The listing builds one solid part. Answer for the finished solid, in the listing's coordinates (mm). Round coordinates to 2 decimals unless told otherwise and drop trailing zeros. Order: outer loops, then holes, each group sorted by start corner. A loop starts at its lowest first (then second) coordinate and runs counter-clockwise, first axis right, second up. Notation, with made-up numbers: (28, 16.25) -> (50, 16.25) arc R14 ccw to (50, 33.25) -> close; hole circle Ø7 at (-22.5, -13). An arc over 180 degrees is marked (long way). Return JSON: item names as keys, results as strings. Group by question number.
(1) This flat-tipped pin is pushed along its axis until it touches: pin 1 (1.5 mm diameter, centred on y = 0.5, z = 18.5, fed in from +X). Where does it stop, or does it pass through?
(2) The part is cut by section A-A (z = 1). Determine the outline of the cut face in (x, y), plus the area to 3 significant figures.
(3) Consider line 1 (X direction, y = 0.85, z = 10); line 2 (Z direction, x = 26.5, y = 0.85). Determine where each line is inside the solid, lowest interval first. Write a range as [from, to].
(4) The part is cut by section B-B (x = 1). Determine the outline of the cut face in (y, z).
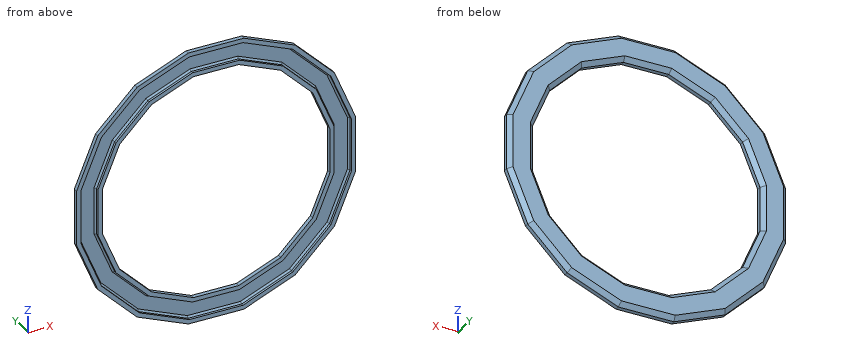
from build123d import *

# Parameters (mm, degrees)
BOSS_EXTRUDE1_DEPTH = 4
CHAMFER1_SIZE       = 2
SHELL1_T            = -2


with BuildPart() as part:
    # Sketch1 → Boss-Extrude1 (new body)
    with BuildSketch(Plane(origin=(0, 0, 0), x_dir=(1, 0, 0), z_dir=(0, 1, 0))):
        Polygon((36.819542328, 55.104339226), (12.92930388, 65), (-12.92930388, 65), (-36.819542328, 55.104339226), (-55.104339226, 36.819542328), (-65, 12.92930388), (-65, -12.92930388), (-55.104339226, -36.819542328), (-36.819542328, -55.104339226), (-12.92930388, -65), (12.92930388, -65), (36.819542328, -55.104339226), (55.104339226, -36.819542328), (65, -12.92930388), (65, 12.92930388), (55.104339226, 36.819542328), align=None)
        Polygon((10.542355471, 53), (-10.542355471, 53), (-30.02208836, 44.931230446), (-44.931230446, 30.02208836), (-53, 10.542355471), (-53, -10.542355471), (-44.931230446, -30.02208836), (-30.02208836, -44.931230446), (-10.542355471, -53), (10.542355471, -53), (30.02208836, -44.931230446), (44.931230446, -30.02208836), (53, -10.542355471), (53, 10.542355471), (44.931230446, 30.02208836), (30.02208836, 44.931230446), align=None, mode=Mode.SUBTRACT)
    extrude(amount=BOSS_EXTRUDE1_DEPTH)

    # Chamfer1
    chamfer1_edges = [part.edges().sort_by_distance(p)[0] for p in [
        (0, 4, -65),
        (-24.874423104, 4, -60.052169613),
        (-45.961940777, 4, -45.961940777),
        (-60.052169613, 4, -24.874423104),
        (-65, 4, 0),
        (-60.052169613, 4, 24.874423104),
        (-45.961940777, 4, 45.961940777),
        (-24.874423104, 4, 60.052169613),
        (0, 4, 65),
        (24.874423104, 4, 60.052169613),
        (45.961940777, 4, -45.961940777),
        (45.961940777, 4, 45.961940777),
        (60.052169613, 4, 24.874423104),
        (20.282221915, 4, -48.965615223),
        (0, 4, -53),
        (-20.282221915, 4, -48.965615223),
        (-37.476659403, 4, -37.476659403),
        (-48.965615223, 4, -20.282221915),
        (-53, 4, 0),
        (-48.965615223, 4, 20.282221915),
        (65, 4, 0),
        (-37.476659403, 4, 37.476659403),
        (-20.282221915, 4, 48.965615223),
        (0, 4, 53),
        (20.282221915, 4, 48.965615223),
        (37.476659403, 4, 37.476659403),
        (48.965615223, 4, 20.282221915),
        (53, 4, 0),
        (48.965615223, 4, -20.282221915),
        (37.476659403, 4, -37.476659403),
        (60.052169613, 4, -24.874423104),
        (24.874423104, 4, -60.052169613),
    ]]
    chamfer(chamfer1_edges, length=CHAMFER1_SIZE)

    # Shell1
    shell1_openings = [part.faces().sort_by_distance(p)[0] for p in [
        (24.170868174, 0, -58.353637759),
    ]]
    offset(amount=SHELL1_T, openings=shell1_openings, kind=Kind.INTERSECTION)


solid = part.part
Answer below:
{
 "1": {"pin 1": "stops at x = 63"},
 "2": {"outline": "(-65, 0) -> (-63, 0) -> (-63, 1.17) -> (-62.17, 2) -> (-55.83, 2) -> (-55, 1.17) -> (-55, 0) -> (-53, 0) -> (-53, 2) -> (-55, 4) -> (-63, 4) -> (-65, 2) -> close; (53, 0) -> (55, 0) -> (55, 1.17) -> (55.83, 2) -> (62.17, 2) -> (63, 1.17) -> (63, 0) -> (65, 0) -> (65, 2) -> (63, 4) -> (55, 4) -> (53, 2) -> close", "area": "57.4 mm²"},
 "3": {"line 1": "x = [-65, -63], [-55, -53], [53, 55], [63, 65]", "line 2": "z = [-59.38, -57.21], [-48.55, -46.39], [46.39, 48.55], [57.21, 59.38]"},
 "4": {"outline": "(0, -65) -> (2, -65) -> (4, -63) -> (4, -55) -> (2, -53) -> (0, -53) -> (0, -55) -> (1.17, -55) -> (2, -55.83) -> (2, -62.17) -> (1.17, -63) -> (0, -63) -> close; (0, 53) -> (2, 53) -> (4, 55) -> (4, 63) -> (2, 65) -> (0, 65) -> (0, 63) -> (1.17, 63) -> (2, 62.17) -> (2, 55.83) -> (1.17, 55) -> (0, 55) -> close"}
}
